```python
from build123d import *

# Parameters (mm, degrees)
SCHNITT_LINEAR_AUSTRAGEN1_DEPTH = 1
LINEAR_AUSTRAGEN1_DEPTH         = 2


with BuildPart() as part:
    # Skizze2 → Rotation1 (revolve)
    with BuildSketch(Plane.XY):
        with BuildLine():
            Line((0, 0), (-1.75, 0))
            Line((-1.75, 0), (-1.75, 0.5))
            Line((-1.75, 0.5), (-1.5, 0.5))
            Line((-1.5, 0.5), (-1.5, 3))
            ThreePointArc((-1.5, 3), (-1.060660172, 4.060660172), (0, 4.5))
            Line((0, 4.5), (0, 0))
        make_face()
    revolve(axis=Axis((0, 0, 0), (0, 1, 0)))

    # Skizze3 → Schnitt-Linear austragen1 (cut)
    with BuildSketch(Plane.XZ):
        with BuildLine():
            Line((1.58113883, -0.75), (1.58113883, 0.75))
            ThreePointArc((1.58113883, 0.75), (1.75, 0), (1.58113883, -0.75))
        make_face()
    extrude(amount=-SCHNITT_LINEAR_AUSTRAGEN1_DEPTH, mode=Mode.SUBTRACT)

    # Skizze4 → Linear austragen1 (add)
    with BuildSketch(Plane.XZ):
        with BuildLine():
            Line((0.6, 0.15), (0.8, 0.15))
            ThreePointArc((0.8, 0.15), (0.870710678, 0.120710678), (0.9, 0.05))
            Line((0.9, 0.05), (0.9, -0.05))
            ThreePointArc((0.9, -0.05), (0.870710678, -0.120710678), (0.8, -0.15))
            Line((0.8, -0.15), (0.6, -0.15))
            ThreePointArc((0.6, -0.15), (0.529289322, -0.120710678), (0.5, -0.05))
            Line((0.5, -0.05), (0.5, 0.05))
            ThreePointArc((0.5, 0.05), (0.529289322, 0.120710678), (0.6, 0.15))
        make_face()
        with BuildLine():
            Line((-0.9, 0.15), (-0.6, 0.15))
            ThreePointArc((-0.6, 0.15), (-0.529289322, 0.120710678), (-0.5, 0.05))
            Line((-0.5, 0.05), (-0.5, -0.05))
            ThreePointArc((-0.5, -0.05), (-0.529289322, -0.120710678), (-0.6, -0.15))
            Line((-0.6, -0.15), (-0.9, -0.15))
            ThreePointArc((-0.9, -0.15), (-0.970710678, -0.120710678), (-1, -0.05))
            Line((-1, -0.05), (-1, 0.05))
            ThreePointArc((-1, 0.05), (-0.970710678, 0.120710678), (-0.9, 0.15))
        make_face()
    extrude(amount=LINEAR_AUSTRAGEN1_DEPTH)


solid = part.part
```
The model under review builds one solid part; all positions refer to its coordinate system, in mm. Coordinates: 2 decimals unless noted, no trailing zeros. Loops run counter-clockwise (first coordinate to the right, second up) from the corner with the lowest first, then second, coordinate; pieces in that order, holes last. Notation, with made-up numbers: (74, 54.5) -> (94, 54.5) arc R16 cw to (94, 62.5) -> close; hole circle Ø11 at (-24.75, 53). An arc over 180 degrees is marked (long way). Answer as CSV lines item,"result".
Item 1: Insertion check: pin 1 (1 mm diameter, centred on y = 3.5, z = 1, fed in from -X); pin 2 (1 mm diameter, centred on x = 1, y = 1.5, fed in from -Z). Each pin has a flat end and moves straight along its axis. Give the tip position at first contact, or say it passes through.
Results below:
pin 1,"stops at x = -1.37"
pin 2,"stops at z = -1.41"
Item 2: Take a section at B-B, the plane y = 2.25. State the section outline as (x, z) points, and give its area (3 significant figures).
Results below:
outline,"circle Ø3 at (0, 0)"
area,"7.07 mm2"
Item 3: For L1, parallel to Y at x = -1.2, z = 1.1; L2, parallel to X at y = 3.5, z = -1.15; L3, parallel to Y at x = -0.55, z = 0.5, list the stretches that pass through material, from the lowest coordinate up.
Results below:
L1,"y = 0 to 0.5"
L2,"x = -0.82 to 0.82"
L3,"y = 0 to 4.3"
Item 4: Take a section at C-C, the plane z = 0.95. State the section outline as (x, y) points, and give its area (3 significant figures).
Results below:
outline,"(-1.47, 0) -> (1.47, 0) -> (1.47, 0.5) -> (1.16, 0.5) -> (1.16, 3) arc R1.16 ccw to (-1.16, 3) -> (-1.16, 0.5) -> (-1.47, 0.5) -> close"
area,"9.39 mm2"
Item 5: Take a section at A-A, the plane x = 0. State the section outline as (y, z) points, and give its area (3 significant figures).
Results below:
outline,"(0, -1.75) -> (0.5, -1.75) -> (0.5, -1.5) -> (3, -1.5) arc R1.5 ccw to (3, 1.5) -> (0.5, 1.5) -> (0.5, 1.75) -> (0, 1.75) -> close"
area,"12.8 mm2"
Item 6: Draft analysis for pull direction Z (two halves, no side actions). For faces 1 (the flat face through (0, 0, 0)), 2 (the cylindrical face through (1.5, 1.77, 0.07)), state which applies: +Z half, -Z half, draft (parallel to the pull), parting line (faces both ways), or undercut.
Results below:
face 1,"draft"
face 2,"parting line"
Item 7: Take a section at D-D, the plane y = 3.5. State the section outline as (x, z) points, and give its area (3 significant figures).
Results below:
outline,"circle Ø2.83 at (0, 0)"
area,"6.28 mm2"
